```python
from build123d import *

# Parameters (mm, degrees)
SKETCH1_R           = 4.085
SKETCH1_R_2         = 5
SKETCH1_R_3         = 2.6
SKETCH1_R_4         = 2.5
SKETCH1_R_5         = 1.75
BOSS_EXTRUDE1_DEPTH = 6
CUT_EXTRUDE1_START  = -1
SKETCH2_R           = 8.085
CUT_EXTRUDE1_DEPTH  = 49.543181614
SKETCH5_R           = 6.75
CUT_EXTRUDE4_DEPTH  = 50.543181614
CHAMFER1_SIZE       = 6
SKETCH6_W           = 11.4
SKETCH6_H           = 12.9
CUT_EXTRUDE5_DEPTH  = 15
SKETCH7_R           = 1.75
SKETCH7_W           = 3
SKETCH7_H           = 5.7
CUT_EXTRUDE6_DEPTH  = 10
CUT_EXTRUDE7_START  = -42
SKETCH8_R           = 1.75
CUT_EXTRUDE7_DEPTH  = 4
CUT_EXTRUDE8_START  = -4
SKETCH8_2_R         = 1.75
CUT_EXTRUDE8_DEPTH  = 4
CHAMFER2_SIZE       = 1


with BuildPart() as part:
    # Sketch1 → Boss-Extrude1 (new body)
    with BuildSketch(Plane.XY):
        with BuildLine():
            Line((-21, -30), (21, -30))
            Line((21, -30), (21, 30))
            Line((21, 30), (-21, 30))
            Line((-21, 30), (-31.4362913, 24.008797289))
            ThreePointArc((-31.4362913, 24.008797289), (-38.93081829, 12.059456115), (-33.194824566, -0.826701779))
            Line((-33.194824566, -0.826701779), (-24, -8))
            Line((-24, -8), (-21, -8))
            Line((-21, -8), (-21, -30))
        make_face()
        with Locations((-10, -23)):
            Circle(SKETCH1_R, mode=Mode.SUBTRACT)
        with Locations((-10, -8)):
            Circle(SKETCH1_R_2, mode=Mode.SUBTRACT)
        with Locations(Location((10, -8, 0), (0, 0, 180))):
            Circle(SKETCH1_R_2, mode=Mode.SUBTRACT)
        with Locations(Location((10, -23, 0), (0, 0, 180))):
            Circle(SKETCH1_R, mode=Mode.SUBTRACT)
        with Locations((-9, 11.974984355)):
            Circle(SKETCH1_R_3, mode=Mode.SUBTRACT)
        with Locations((-23.968279978, 11)):
            Circle(SKETCH1_R_4, mode=Mode.SUBTRACT)
        with Locations((16, 27)):
            Circle(SKETCH1_R_5, mode=Mode.SUBTRACT)
        with Locations((-8, 27)):
            Circle(SKETCH1_R_5, mode=Mode.SUBTRACT)
    extrude(amount=BOSS_EXTRUDE1_DEPTH)

    # Sketch2 → Cut-Extrude1 (cut, through all)
    with BuildSketch(Plane.XY.offset(6).offset(CUT_EXTRUDE1_START)):
        with Locations((-10, -8)):
            Circle(SKETCH2_R)
        with Locations(Location((10, -8, 0), (0, 0, 180))):
            Circle(SKETCH2_R)
    extrude(amount=-CUT_EXTRUDE1_DEPTH, mode=Mode.SUBTRACT)

    # Sketch5 → Cut-Extrude4 (cut, through all)
    with BuildSketch(Plane.XY.offset(6)):
        with Locations((-23.968279978, 11)):
            Circle(SKETCH5_R)
    extrude(amount=-CUT_EXTRUDE4_DEPTH, mode=Mode.SUBTRACT)

    # Chamfer1
    # the kernel refuses this chamfer: 6 mm, written as the material it takes off along each edge
    with BuildSketch(Plane(origin=(-36.430097928, -30, 0), x_dir=(0, 0.9996219169112969, -0.027495876610586382), z_dir=(1, 0, 0))) as chamfer1_piece_1:
        Polygon((CHAMFER1_SIZE * 0.999621916911, CHAMFER1_SIZE * 0.0274958766106), (-CHAMFER1_SIZE * 0.0274958766106, CHAMFER1_SIZE * 0.999621916911), (0, 0), align=None)
    extrude(amount=72.860195856, mode=Mode.SUBTRACT)

    # Sketch6 → Cut-Extrude5 (cut)
    with BuildSketch(Plane(origin=(0, 0, 0), x_dir=(-1, 0, 0), z_dir=(0, 0, -1))):
        with Locations((-15.3, 7.55)):
            Rectangle(SKETCH6_W, SKETCH6_H)
    extrude(amount=-CUT_EXTRUDE5_DEPTH, mode=Mode.SUBTRACT)

    # Sketch7 → Cut-Extrude6 (cut)
    with BuildSketch(Plane(origin=(0, 0, 0), x_dir=(-1, 0, 0), z_dir=(0, 0, -1))):
        with Locations((23.968279978, 23.5)):
            Circle(SKETCH7_R)
        with Locations((23.968279978, -1.5)):
            Circle(SKETCH7_R)
        with Locations((-18.5, -16)):
            Rectangle(SKETCH7_W, SKETCH7_H)
        with Locations((18.5, -16)):
            Rectangle(SKETCH7_W, SKETCH7_H)
        with Locations((-18.5, 19)):
            Rectangle(SKETCH7_W, SKETCH7_H)
    extrude(amount=-CUT_EXTRUDE6_DEPTH, mode=Mode.SUBTRACT)

    # Sketch8 → Cut-Extrude7 (cut)
    with BuildSketch(Plane(origin=(21, 0, 0), x_dir=(0, 0, -1), z_dir=(1, 0, 0)).offset(CUT_EXTRUDE7_START)):
        with Locations(Location((-3, -16, 0), (0, 0, 270))):
            Circle(SKETCH8_R)
        with Locations(Location((-3, 19, 0), (0, 0, 90))):
            Circle(SKETCH8_R)
    extrude(amount=CUT_EXTRUDE7_DEPTH, mode=Mode.SUBTRACT)

    # Sketch8<2> → Cut-Extrude8 (cut)
    with BuildSketch(Plane(origin=(21, 0, 0), x_dir=(0, 0, -1), z_dir=(1, 0, 0)).offset(CUT_EXTRUDE8_START)):
        with Locations(Location((-3, -16, 0), (0, 0, 270))):
            Circle(SKETCH8_2_R)
        with Locations(Location((-3, 19, 0), (0, 0, 90))):
            Circle(SKETCH8_2_R)
    extrude(amount=CUT_EXTRUDE8_DEPTH, mode=Mode.SUBTRACT)

    # Chamfer2
    chamfer2_edges = [part.edges().sort_by_distance(p)[0] for p in [
        (-30.718279978, 11, 6),
    ]]
    chamfer(chamfer2_edges, length=CHAMFER2_SIZE)


solid = part.part
```
Model file for the job. Use its own axes, mm. A direction names the side the tool comes from. Coordinates: 2 decimals unless noted, no trailing zeros. Write each loop counter-clockwise with the first axis right and the second up, starting at its lowest first coordinate (ties: lowest second). Pieces come first, ordered by that corner, then holes. Notation, with made-up numbers: (41, -26) - (86, -26) arc R26 cw to (86, -2) - close; hole circle Ø6 at (19, 20). An arc over 180 degrees is marked (long way). Use a Markdown table: item, result. Add a question column.
Item 1: 3-axis set-ups, long thin cutter, end or side, ignore diameter. For faces 4 (the face through (15.959, -13.464, 2.535)), 5 (the face through (20, -17.3, 1.6)), 6 (the face through (9.6, 7, 3)), 7 (the face through (-28.662, -4.363, 2.958)), 8 (the face through (20.49, 17.25, 3.08)): which of +Z, -Z, +X, -X, +Y, -Y reach the whole face in a straight line?
Item 2: Two-plate mould, pull along Z, no slides. Class faces 1 (the face through (-3, 0, 6)), 2 (the face through (-21, -19, 3)), 3 (the face through (-19.03, 17.25, 3.08)): pulls with the +Z half, pulls with the -Z half, needs draft (parallel to the pull), parting line crosses it, or undercut.
Item 3: Band-saw the part on B-B, the plane x = -9. Write the cut outline in (y, z), and give its area (3 significant figures).
Item 4: Band-saw the part on A-A, the plane y = -23. Write the cut outline in (x, z) (3 decimals).
Item 5: Drill centre lines: line 1 along X through (y, z) = (-23, 5.5) (3 decimals); line 2 along Y through (x, z) = (10, 1.6) (3 decimals); line 3 along X through (y, z) = (-15, 3.95). Where is each one in solid material? Low to high.
Item 6: Band-saw the part on D-D, the plane y = -15. Write the cut outline in (x, z).
Item 7: Drop flat-ended pins along their axis: pin 1 (13 mm diameter, centred on x = 10, y = -8, fed in from -Z); pin 2 (3 mm diameter, centred on y = -12, z = 3.5, fed in from -X); pin 3 (3 mm diameter, centred on y = -16, z = 3, fed in from -X). Give the stop position or say it passes through.
Item 8: Band-saw the part on C-C, the plane x = 16. Write the cut outline in (y, z).
A:
| question | item | result |
|---|---|---|
| 1 | face 4 | -Z |
| 1 | face 5 | +Z, -Z |
| 1 | face 6 | +Z, -Z, +X |
| 1 | face 7 | +Z, -Z, -X, -Y |
| 1 | face 8 | +X |
| 2 | face 1 | pulls with the +Z half |
| 2 | face 2 | needs draft |
| 2 | face 3 | undercut |
| 3 | outline | (-30, 6) - (-26.96, 2.96) - (-26.96, 6) - close; (-19.04, 0) - (-16.02, 0) - (-16.02, 5) - (-12.9, 5) - (-12.9, 6) - (-19.04, 6) - close; (-3.1, 5) - (0.02, 5) - (0.02, 0) - (9.37, 0) - (9.37, 6) - (-3.1, 6) - close; (14.57, 0) - (25.56, 0) - (25.56, 6) - (14.57, 6) - close; (28.44, 0) - (30, 0) - (30, 6) - (28.44, 6) - close |
| 3 | area | 160 mm² |
| 4 | outline | (-21, 0) - (-14.085, 0) - (-14.085, 6) - (-21, 6) - close; (-5.915, 0) - (5.915, 0) - (5.915, 6) - (-5.915, 6) - close; (14.085, 0) - (21, 0) - (21, 6) - (14.085, 6) - close |
| 5 | line 1 | x = -21 to -14.085, -5.915 to 5.915, 14.085 to 21 |
| 5 | line 2 | y = -18.915 to -16.085, 0.085 to 1.1, 14 to 30 |
| 5 | line 3 | x = -17 to -14.05, -5.95 to 5.95, 14.05 to 17 |
| 6 | outline | (-21, 0) - (-20, 0) - (-20, 1.56) - (-21, 1.56) - close; (-21, 4.44) - (-20, 4.44) - (-20, 6) - (-21, 6) - close; (-17, 0) - (-14.05, 0) - (-14.05, 5) - (-5.95, 5) - (-5.95, 0) - (5.95, 0) - (5.95, 5) - (14.05, 5) - (14.05, 0) - (17, 0) - (17, 6) - (-17, 6) - close; (20, 0) - (21, 0) - (21, 1.56) - (20, 1.56) - close; (20, 4.44) - (21, 4.44) - (21, 6) - (20, 6) - close |
| 7 | pin 1 | stops at z = 5 |
| 7 | pin 2 | stops at x = -21 |
| 7 | pin 3 | stops at x = -17 |
| 8 | outline | (-30, 6) - (-24, 0) - (-13.42, 0) - (-13.42, 5) - (-2.58, 5) - (-2.58, 0) - (1.1, 0) - (1.1, 6) - close; (14, 0) - (25.25, 0) - (25.25, 6) - (14, 6) - close; (28.75, 0) - (30, 0) - (30, 6) - (28.75, 6) - close |
